Geometry check sheet. Reference: the model listing, model coordinates, mm. A direction names the side the tool comes from. Round coordinates to 2 decimals unless told otherwise and drop trailing zeros. Loops run counter-clockwise (first coordinate to the right, second up) from the corner with the lowest first, then second, coordinate; pieces in that order, holes last. Notation, with made-up numbers: M 20.25,67.25 L 66.25,67.25 A17 cw 66.25,77.25 Z; hole C 13,67.5 d6. An arc over 180 degrees is marked long. Write item = value, one per line.
Autodesk Inventor part; units mm, degrees
ref_plane "YZ Plane" through (0, 0, 0) normal (1, 0, 0) x (0, 1, 0)
ref_plane "XZ Plane" through (0, 0, 0) normal (0, 1, 0) x (-1, 0, 0)
ref_plane "XY Plane" through (0, 0, 0) normal (0, 0, 1) x (1, 0, 0)
sketch "Esboço1" plane through (0, 0, 0) normal (0, 1, 0) x (-1, 0, 0)
  line L0 (9.525, 38.1) -> (-9.525, 38.1)
  line L1 (-9.525, 38.1) -> (-9.525, -38.1)
  line L2 (-9.525, -38.1) -> (9.525, -38.1)
  line L3 (9.525, -38.1) -> (9.525, 38.1)
  line L4 (9.525, 38.1) -> (-9.525, -38.1) construction
  line L5 (-9.525, 38.1) -> (9.525, -38.1) construction
  line L6 (0, -53.7953) -> (0, 49.8481)
  line L7 (-9.525, -38.1) -> (-9.525, -19.04) construction
  line L8 (-9.525, -19.04) -> (-9.525, 38.1) construction
  line L9 (0, -38.1) -> (0, -30.1) construction
  line L10 (0, 38.1) -> (0, 30.1) construction
  circle A0 centre (0, 30.1) radius 2.39
  arc A1 (4.205, -34.8582) -> (-4.205, -34.8582) centre (0, -30.1) ccw
  line L11 (-4.205, -34.8582) -> (4.205, -34.8582)
  point P0 (0, 0)
  dimension "d0" = 19.05
  dimension "d4" = 76.2
  dimension "d5" = 8
  dimension "d8" = 4.78
  dimension "d9" = 12.7
extrude "Extrusão1" add sketch "Esboço1" along normal blind 6.35 contours L3 L2 L6 L11 A1 A0 L0 | L6 A0 A1 L11 L2 L1 L0
properties part number "Virabrequim8"
(1) Sectioned sample at C-C on x = 0. Record the cut outline in (y, z), then the cut area to 3 significant figures.
Result set:
outline = M 0,-38.1 L 6.35,-38.1 L 6.35,-34.86 L 0,-34.86 Z; M 0,-23.75 L 6.35,-23.75 L 6.35,27.71 L 0,27.71 Z; M 0,32.49 L 6.35,32.49 L 6.35,38.1 L 0,38.1 Z
area = 383 mm2
(2) Material ranges on line 1 along Z through (x, y) = (0, 3.5); line 2 along X through (y, z) = (3.5, -30.1) (3 decimals); line 3 along X through (y, z) = (2.75, 30.1) (3 decimals), recorded low to high. Write a range as from..to.
Result set:
line_1 = -38.1..-34.86, -23.75..27.71, 32.49..38.1
line_2 = -9.525..-6.35, 6.35..9.525
line_3 = -9.525..-2.39, 2.39..9.525
(3) Depth check by flat-ended pin: pin 1 Ø7.5 at (x, z) = (0, 30.1) entering from -Y. Enter the tip coordinate at first touch or a pass-through.
Result set:
pin_1 = 0
(4) Tool access check on faces 4 (the flat face through (0, 3, -34.858)), 5 (the flat face through (0, 6.35, 1)). Record the directions out of +Z, -Z, +X, -X, +Y, -Y that give a thin tool (end or side, any length) a straight path to the whole face; none if there is none.
Result set:
face_4 = +Y, -Y
face_5 = +Z, -Z, +X, -X, +Y
(5) Sectioned sample at D-D on x = 5.5. Record the cut outline in (y, z).
Result set:
outline = M 0,-38.1 L 6.35,-38.1 L 6.35,-33.27 L 0,-33.27 Z; M 0,-26.93 L 6.35,-26.93 L 6.35,38.1 L 0,38.1 Z
(6) Release check for a two-part mould opening along Z. For faces 1 (the flat face through (-9.525, 3, -1)), 2 (the cylindrical face through (0.215, 3.131, -23.754)), 3 (the flat face through (0, 3, -38.1)) record: released by +Z, released by -Z, zero draft, split by the parting line, or undercut.
Result set:
face_1 = zero draft
face_2 = undercut
face_3 = released by -Z
(7) Sectioned sample at A-A on z = 30.1. Record the cut outline in (x, y) (3 decimals), then the cut area to 3 significant figures.
Result set:
outline = M -9.525,0 L -2.39,0 L -2.39,6.35 L -9.525,6.35 Z; M 2.39,0 L 9.525,0 L 9.525,6.35 L 2.39,6.35 Z
area = 90.6 mm2
(8) Sectioned sample at B-B on y = 5.25. Record the cut outline in (x, z) (3 decimals), then the cut area to 3 significant figures.
Result set:
outline = M -9.525,-38.1 L 9.525,-38.1 L 9.525,38.1 L -9.525,38.1 Z; hole M -4.205,-34.858 L 4.205,-34.858 A6.35 ccw long Z; hole C 0,30.1 d4.78
area = 1,320 mm2
